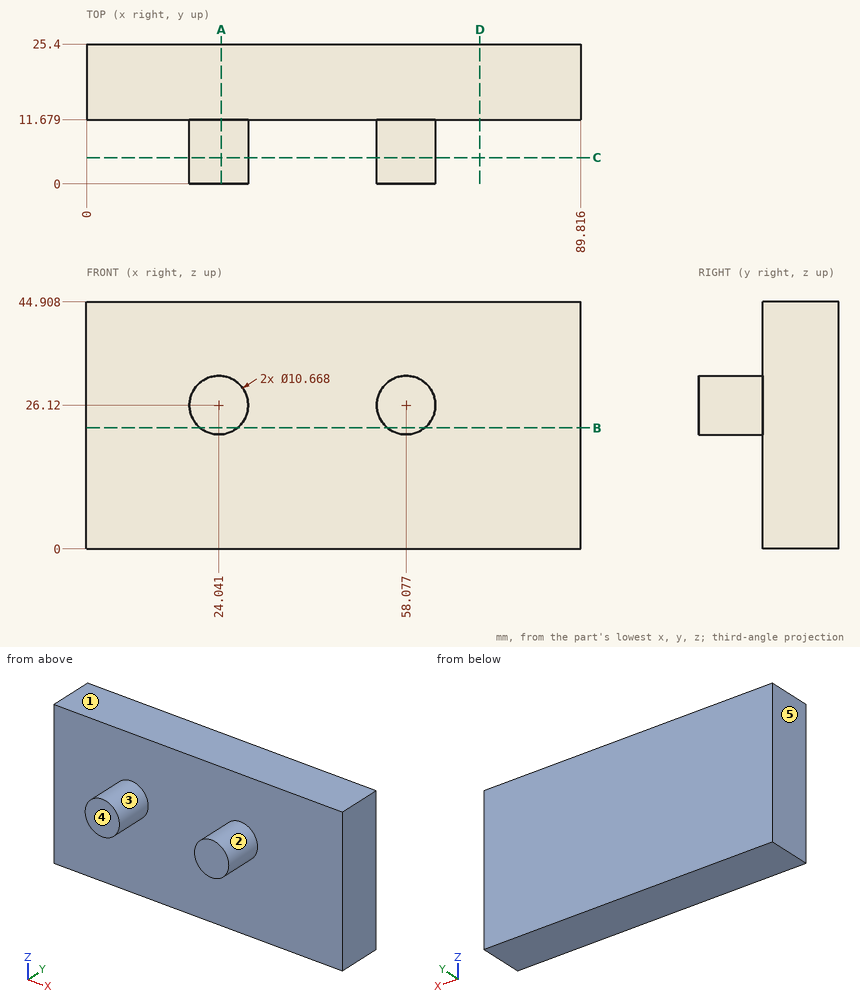
Could you check a few things on this drawing? It's one solid part, dimensions in mm from its lowest x, y, z. A direction names the side the tool comes from. Give positions to 0.01 mm unless a question says otherwise; leave off trailing zeros. Order: outer loops, then holes, each group sorted by start corner. A loop starts at its lowest first (then second) coordinate and runs counter-clockwise, first axis right, second up. Notation, with made-up numbers: (11, 79.5) -> (53, 79.5) arc R26 ccw to (53, 97.5) -> close; hole circle Ø4 at (-11, 34.25). An arc over 180 degrees is marked (long way). Answer in a Markdown table with one row per item. Add a question column.
Item 1: Please list where these lines run through material, in increasing order: probe 1 along Y at (x, z) = (34.5, 7.5); probe 2 along Z at (x, y) = (60, 2.25) (1 decimal); probe 3 along Z at (x, y) = (22, 4.25).
Item 2: We'd pull the mould along X, two halves only. Please class the marked faces 3, 4 and 5: pulls with the +X half, pulls with the -X half, needs draft (parallel to the pull), parting line crosses it, or undercut.
Item 3: For the marked faces 1 and 2, which set-ups out of +Z, -Z, +X, -X, +Y, -Y let a thin tool reach every point of the face, with its end or its side?
Item 4: Imagine slicing it at C-C (y = 4.75). List the corners of the cut face in (x, z) for me (1 decimal).
Item 5: Imagine slicing it at A-A (x = 24.5). List the corners of the cut face in (y, z) for me (1 decimal), and give its area (3 significant figures).
Item 6: Imagine slicing it at D-D (x = 71.5). List the corners of the cut face in (y, z) for me.
Item 7: I'm going to push a flat-ended pin straight in: P1, Ø3, axis at x = 47.5, z = 29.5, coming from the -Y side. Where does the tip first touch, or does it pass through?
Item 8: Imagine slicing it at B-B (z = 22). List the corners of the cut face in (x, y) for me (1 decimal).
Result:
| question | item | result |
|---|---|---|
| 1 | probe 1 | 11.68 to 25.4 |
| 1 | probe 2 | 21.1 to 31.1 |
| 1 | probe 3 | 21.19 to 31.05 |
| 2 | face 3 | undercut |
| 2 | face 4 | needs draft |
| 2 | face 5 | pulls with the -X half |
| 3 | face 1 | +Z, +X, -X, +Y, -Y |
| 3 | face 2 | -Y |
| 4 | outline | circle Ø10.7 at (24, 26.1); circle Ø10.7 at (58.1, 26.1) |
| 5 | outline | (0, 20.8) -> (11.7, 20.8) -> (11.7, 0) -> (25.4, 0) -> (25.4, 44.9) -> (11.7, 44.9) -> (11.7, 31.4) -> (0, 31.4) -> close |
| 5 | area | 740 mm2 |
| 6 | outline | (11.68, 0) -> (25.4, 0) -> (25.4, 44.91) -> (11.68, 44.91) -> close |
| 7 | P1 | y = 11.68 |
| 8 | outline | (0, 11.7) -> (20.7, 11.7) -> (20.7, 0) -> (27.4, 0) -> (27.4, 11.7) -> (54.7, 11.7) -> (54.7, 0) -> (61.5, 0) -> (61.5, 11.7) -> (89.8, 11.7) -> (89.8, 25.4) -> (0, 25.4) -> close |
